from build123d import *

# Parameters (mm, degrees)
SKETCH1_R                = 50.8
SKETCH1_R_2              = 48.26
COUPLER_EXTRUSION_DEPTH  = 508
BULKHEAD_HOLE_REACH      = 522.545
BULKHEAD_HOLE_END_RADIUS = 48.26
SKETCH2_R                = 1.6383
CIRPATTERN1_COUNT        = 4
CUT_EXTRUDE1_REACH       = 522.545
CUT_EXTRUDE1_END_RADIUS  = 48.26
SKETCH3_R                = 1.7526
CIRPATTERN2_COUNT        = 4


with BuildPart() as part:
    # Sketch1 → Coupler Extrusion (new body)
    with BuildSketch(Plane(origin=(0, 0, 0), x_dir=(1, 0, 0), z_dir=(0, 1, 0))):
        Circle(SKETCH1_R)
        Circle(SKETCH1_R_2, mode=Mode.SUBTRACT)
    extrude(amount=COUPLER_EXTRUSION_DEPTH)

    # Bulkhead Hole: up to this cylinder (the profile starts outside it)
    bulkhead_hole_end = Plane(origin=(0, 336.55, 0), z_dir=(0, -1, 0)) * Cylinder(BULKHEAD_HOLE_END_RADIUS, 1142.61, mode=Mode.PRIVATE)
    # Sketch2 → Bulkhead Hole (cut, up to the surface)
    with BuildSketch(Plane.XY.offset(50.8), mode=Mode.PRIVATE) as bulkhead_hole_sk1:
        with Locations((0, 336.55)):
            Circle(SKETCH2_R)
    bulkhead_hole_tool1 = extrude(bulkhead_hole_sk1.sketch, amount=-BULKHEAD_HOLE_REACH, mode=Mode.PRIVATE) - bulkhead_hole_end
    bulkhead_hole = bulkhead_hole_tool1.solids().sort_by_distance((0, 336.55, 50.8))[0]
    add(bulkhead_hole, mode=Mode.SUBTRACT)

    # CirPattern1: Bulkhead Hole ×4 about axis
    cirpattern1_axis = Axis((0, 508, 0), (0, -1, 0))
    for i in range(1, CIRPATTERN1_COUNT):
        add(bulkhead_hole.rotate(cirpattern1_axis, i * 360 / CIRPATTERN1_COUNT), mode=Mode.SUBTRACT)

    # Cut-Extrude1: up to this cylinder (the profile starts outside it)
    cut_extrude1_end = Plane(origin=(0, 196.85, 0), z_dir=(0, -1, 0)) * Cylinder(CUT_EXTRUDE1_END_RADIUS, 1142.61, mode=Mode.PRIVATE)
    # Sketch3 → Cut-Extrude1 (cut, up to the surface)
    with BuildSketch(Plane.XY.offset(50.8), mode=Mode.PRIVATE) as cut_extrude1_sk1:
        with Locations((0, 196.85)):
            Circle(SKETCH3_R)
    cut_extrude1_tool1 = extrude(cut_extrude1_sk1.sketch, amount=-CUT_EXTRUDE1_REACH, mode=Mode.PRIVATE) - cut_extrude1_end
    cut_extrude1 = cut_extrude1_tool1.solids().sort_by_distance((0, 196.85, 50.8))[0]
    add(cut_extrude1, mode=Mode.SUBTRACT)

    # CirPattern2: Cut-Extrude1 ×4 about axis
    cirpattern2_axis = Axis((0, 508, 0), (0, -1, 0))
    for i in range(1, CIRPATTERN2_COUNT):
        add(cut_extrude1.rotate(cirpattern2_axis, i * 360 / CIRPATTERN2_COUNT), mode=Mode.SUBTRACT)


solid = part.part
Work out the finished part from the listing and answer in its coordinate system (mm). Round coordinates to 2 decimals unless told otherwise and drop trailing zeros. Write each loop counter-clockwise with the first axis right and the second up, starting at its lowest first coordinate (ties: lowest second). Pieces come first, ordered by that corner, then holes. Notation, with made-up numbers: M -16,74 L 26,74 A7 ccw 26,79 Z; hole C -7.75,53.5 d5. An arc over 180 degrees is marked long. Use a Markdown table: item, result.
1) The part is cut by section A-A on z = -34.5. Give the vertices of the cut face in (x, y), plus the area to 3 significant figures.
Taken from the geometry:
| item | result |
|---|---|
| outline | M -37.29,0 L -33.75,0 L -33.75,508 L -37.29,508 Z; M 33.75,0 L 37.29,0 L 37.29,508 L 33.75,508 Z |
| area | 3,600 mm2 |
2) The part is cut by section C-C on y = 162. Give the vertices of the cut face in (x, z), plus the area to 3 significant figures.
Taken from the geometry:
| item | result |
|---|---|
| outline | C 0,0 d101.6; hole C 0,0 d96.52 |
| area | 790 mm2 |
3) Flat-ended cylindrical pins translate along their axes: pin 1 (4 mm diameter, centred on y = 337.5, z = -29.5, fed in from +X); pin 2 (5.5 mm diameter, centred on y = 196.85, z = 0, fed in from -X); pin 3 (10 mm diameter, centred on x = -40.5, y = 302.5, fed in from +Z); pin 4 (1 mm diameter, centred on x = -2.5, y = 139, fed in from +Z). Find the tip coordinate at first contact, or state that the pin passes through.
Taken from the geometry:
| item | result |
|---|---|
| pin 1 | stops at x = 42.71 |
| pin 2 | stops at x = -50.8 |
| pin 3 | stops at z = 36.34 |
| pin 4 | stops at z = 50.76 |
4) The part is cut by section B-B on x = 14.5. Give the vertices of the cut face in (y, z).
Taken from the geometry:
| item | result |
|---|---|
| outline | M 0,-48.69 L 508,-48.69 L 508,-46.03 L 0,-46.03 Z; M 0,46.03 L 508,46.03 L 508,48.69 L 0,48.69 Z |
5) Consider line 1 (Y direction, x = -49.5, z = 0); line 2 (Z direction, x = 2, y = 439.5); line 3 (Z direction, x = -4, y = 102.5). Determine where each line is inside the solid, lowest interval first. Write a range as [from, to].
Taken from the geometry:
| item | result |
|---|---|
| line 1 | y = [0, 195.1], [198.6, 334.91], [338.19, 508] |
| line 2 | z = [-50.76, -48.22], [48.22, 50.76] |
| line 3 | z = [-50.64, -48.09], [48.09, 50.64] |
6) Determine the mould class of faces 1 (the face through (45, 508, 19)), 2 (the face through (44.58, 250.44, 18.48)), 3 (the face through (-11.012, 250.444, 49.592)) for opening direction Z: pulls with the +Z half, pulls with the -Z half, needs draft (parallel to the pull), parting line crosses it, or undercut.
Taken from the geometry:
| item | result |
|---|---|
| face 1 | needs draft |
| face 2 | undercut |
| face 3 | parting line crosses it |
